```python
from build123d import *


with BuildPart() as part:
    # Schizzo1 → Rivoluzione1 (revolve)
    with BuildSketch(Plane.XY, mode=Mode.PRIVATE) as rivoluzione1_sk:
        Polygon((6.830726988, -8.387277259), (5.972508756, -5.587032245), (5.05357518, -4.82347792), (4.432541097, 8.217841328), (0, 8.217841328), (0, 8.917841328), (5.1, 8.917841328), (5.738114638, -4.482158672), (6.580560922, -5.182158672), (7.5, -8.182158672), align=None)
    revolve(rivoluzione1_sk.sketch.rotate(Axis((0, 55, 0), (0, -1, 0)), 90), axis=Axis((0, 55, 0), (0, -1, 0)))


solid = part.part
```
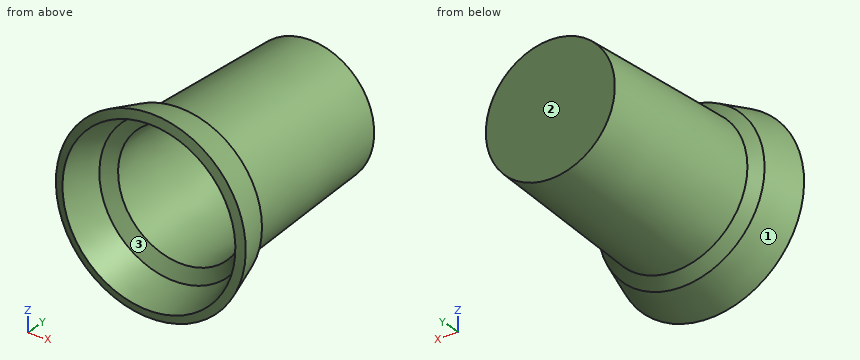
Verification items for the finished model (mm, model axes). Face numbers are marked on the shaded views. Give positions to 0.01 mm unless a question says otherwise; leave off trailing zeros. Write each loop counter-clockwise with the first axis right and the second up, starting at its lowest first coordinate (ties: lowest second). Pieces come first, ordered by that corner, then holes. Notation, with made-up numbers: M 25,-11.5 L 33,-11.5 A25 cw 33,26.5 Z; hole C -12,-9 d10. An arc over 180 degrees is marked long. One line per question, with ' | ' between items.
1) Section check A-A on x = 0. Enter the section's corners in (y, z).
Result:
outline: M -8.39,-6.83 L -8.18,-7.5 L -5.18,-6.58 L -4.48,-5.74 L 8.92,-5.1 L 8.92,5.1 L -4.48,5.74 L -5.18,6.58 L -8.18,7.5 L -8.39,6.83 L -5.59,5.97 L -4.82,5.05 L 8.22,4.43 L 8.22,-4.43 L -4.82,-5.05 L -5.59,-5.97 Z
2) Thickness scan on line 1 along Z through (x, y) = (2.5, 6.5); line 2 along Z through (x, y) = (2.75, 0.5); line 3 along Y through (x, z) = (-1, -2.75). Record the ranges inside material, lowest first. Write a range as [from, to].
Result:
line 1: z = [-4.58, -3.76], [3.76, 4.58] | line 2: z = [-4.76, -3.93], [3.93, 4.76] | line 3: y = [8.22, 8.92]
3) Section check C-C on y = -6.75. Enter the section's corners in (x, z), plus the area to 3 significant figures.
Result:
outline: C 0,0 d14.12; hole C 0,0 d12.66 | area: 30.8 mm2
4) Gauge pin test, flat ends, axial feed: pin 1 Ø3 at (x, y) = (-6, -4.5) entering from -Z; pin 2 Ø1.5 at (y, z) = (5.5, 4.5) entering from +X; pin 3 Ø3 at (x, y) = (1.5, 3.5) entering from -Z. Record the tip position at first contact, or that the pin passes through.
Result:
pin 1: stops at z = -4.64 | pin 2: stops at x = 3.69 | pin 3: stops at z = -5.39
5) Section check D-D on y = -0.5. Enter the section's corners in (x, z), plus the area to 3 significant figures.
Result:
outline: C 0,0 d11.1; hole C 0,0 d9.7 | area: 22.9 mm2
6) Section check B-B on z = 0. Enter the section's corners in (x, y), plus the area to 3 significant figures.
Result:
outline: M -7.5,-8.18 L -6.83,-8.39 L -5.97,-5.59 L -5.05,-4.82 L -4.43,8.22 L 4.43,8.22 L 5.05,-4.82 L 5.97,-5.59 L 6.83,-8.39 L 7.5,-8.18 L 6.58,-5.18 L 5.74,-4.48 L 5.1,8.92 L -5.1,8.92 L -5.74,-4.48 L -6.58,-5.18 Z | area: 31.1 mm2
7) Mould release check, pull along Z, two halves, no side actions. Record for the marked faces 1, 2 and 3: released by +Z, released by -Z, zero draft, split by the parting line, or undercut.
Result:
face 1: split by the parting line | face 2: zero draft | face 3: undercut
